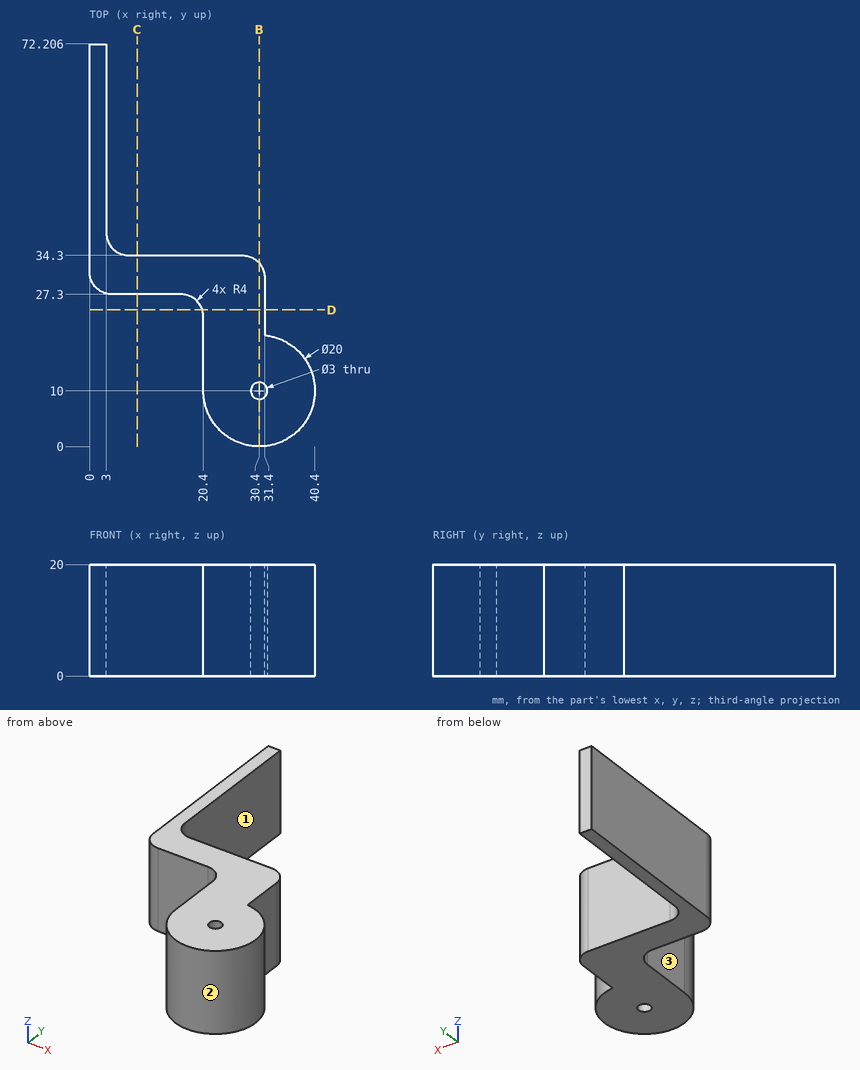
The figure shows three views and two pictorial views of one solid part (mm, origin at its lowest corner). Answer the questions. A direction names the side the tool comes from. Coordinates: 2 decimals unless noted, no trailing zeros. Loops run counter-clockwise (first coordinate to the right, second up) from the corner with the lowest first, then second, coordinate; pieces in that order, holes last. Notation, with made-up numbers: (88, 60) -> (129, 60) arc R30 cw to (129, 93) -> close; hole circle Ø4 at (54, 89). An arc over 180 degrees is marked (long way). Write item = value, one per line. Start each with the question number.
1) A tool of negligible diameter and unlimited length cuts with its end or side. For the marked faces 1, 2 and 3, from which of +Z, -Z, +X, -X, +Y, -Y can it reach the whole face along a straight path? Write none if from no direction.
2) A cutting plane is placed at D-D (y = 24.5). Give the vertices of the cut face in (x, z) (1 decimal).
3) Straight lines are drawn through the part: line 1 (X direction, y = 10, z = 8.75); line 2 (X direction, y = 66, z = 3); line 3 (Y direction, x = 31, z = 16.75) (1 decimal). For each, find the intervals that lie inside material, in ascending order. Write a range as from..to.
4) Given pin 1 Ø1 at (y, z) = (12.5, 4) entering from +X; pin 2 Ø1 at (y, z) = (42.5, 9.5) entering from +X; pin 3 Ø8 at (x, z) = (15.5, 17) entering from +Y; pin 4 Ø1.8 at (x, y) = (30.4, 10) entering from -Z, each flat-ended and moving along its own axis, determine where each tip first touches the part or whether it passes through.
5) A cutting plane is placed at B-B (x = 30.4). Give the vertices of the cut face in (y, z) (1 decimal), then the cut area to 3 significant figures.
6) A cutting plane is placed at C-C (x = 8.5). Give the vertices of the cut face in (y, z), then the cut area to 3 significant figures.
Responses:
q1.face_1 = +Z, -Z, +X, +Y
q1.face_2 = +Z, -Z
q1.face_3 = +Z, -Z, -X, -Y
q2.outline = (20.2, 0) -> (31.4, 0) -> (31.4, 20) -> (20.2, 20) -> close
q3.line_1 = 20.4..28.9, 31.9..40.4
q3.line_2 = 0..3
q3.line_3 = 0..8.6, 11.4..32
q4.pin_1 = 40.2
q4.pin_2 = 3
q4.pin_3 = 34.3
q4.pin_4 = through
q5.outline = (0, 0) -> (8.5, 0) -> (8.5, 20) -> (0, 20) -> close; (11.5, 0) -> (32.9, 0) -> (32.9, 20) -> (11.5, 20) -> close
q5.area = 599 mm²
q6.outline = (27.3, 0) -> (34.3, 0) -> (34.3, 20) -> (27.3, 20) -> close
q6.area = 140 mm²
